Geometry check sheet. Reference: the model listing, model coordinates, mm. A direction names the side the tool comes from. Give positions to 0.01 mm unless a question says otherwise; leave off trailing zeros. Loops run counter-clockwise (first coordinate to the right, second up) from the corner with the lowest first, then second, coordinate; pieces in that order, holes last. Notation, with made-up numbers: (88, 0.5) -> (122, 0.5) arc R16 cw to (122, 4.5) -> close; hole circle Ø10 at (-26.5, 58.25). An arc over 180 degrees is marked (long way). Write item = value, one per line.
Autodesk Inventor part; units mm, degrees
ref_plane "YZ Plane" through (0, 0, 0) normal (1, 0, 0) x (0, 1, 0)
ref_plane "XZ Plane" through (0, 0, 0) normal (0, 1, 0) x (-1, 0, 0)
ref_plane "XY Plane" through (0, 0, 0) normal (0, 0, 1) x (1, 0, 0)
sketch "Skizze1" plane through (0, 0, 0) normal (0, 0, 1) x (1, 0, 0)
  circle A0 centre (0, 0) radius 4
  dimension "d0" = 8
extrude "Extrusion1" add sketch "Skizze1" along normal blind 40
sketch "Skizze2" plane through (0, 0, 0) normal (0, 0, -1) x (-1, 0, 0)
  circle A0 centre (0, 0) radius 3.5
  dimension "d3" = 7
extrude "Extrusion2" add sketch "Skizze2" along normal blind 5
thread "Gewinde1"
sketch "Skizze3" plane through (0, 0, 40) normal (0, 0, 1) x (1, 0, 0)
  circle A0 centre (0, 0) radius 3.5
  dimension "d8" = 7
extrude "Extrusion3" add sketch "Skizze3" along normal blind 7
properties part number "M8 inductive probe"
Item 1: Section check A-A, the plane y = 0. Record the cut outline in (x, z).
Answer:
outline = (-4, 0) -> (-3.5, 0) -> (-3.5, -5) -> (3.5, -5) -> (3.5, 0) -> (4, 0) -> (4, 40) -> (3.5, 40) -> (3.5, 47) -> (-3.5, 47) -> (-3.5, 40) -> (-4, 40) -> close
Item 2: Tool access check on faces 1 (the cylindrical face through (3.233, 1.341, 43.451)), 2 (the cylindrical face through (-3.233, 1.341, -2.465)), 3 (the cylindrical face through (-0.867, 3.905, 19.72)). Record the directions out of +Z, -Z, +X, -X, +Y, -Y that give a thin tool (end or side, any length) a straight path to the whole face; none if there is none.
Answer:
face_1 = +Z
face_2 = -Z
face_3 = +Z, -Z
Item 3: Section check C-C, the plane z = 29.5. Record the cut outline in (x, y), plus the area to 3 significant figures.
Answer:
outline = circle Ø8 at (0, 0)
area = 50.3 mm^2
Item 4: Section check D-D, the plane z = -1. Record the cut outline in (x, y), plus the area to 3 significant figures.
Answer:
outline = circle Ø7 at (0, 0)
area = 38.5 mm^2
Item 5: Gauge pin test, flat ends, axial feed: pin 1 (1.5 mm diameter, centred on x = 3, z = 26.5, fed in from +Y); pin 2 (1.5 mm diameter, centred on x = -3, y = 2.5, fed in from -Z); pin 3 (1.5 mm diameter, centred on y = -2.5, z = 2, fed in from -X); pin 4 (1.5 mm diameter, centred on y = -1.5, z = 8.5, fed in from -X). Record the tip position at first contact, or that the pin passes through.
Answer:
pin_1 = 3.31
pin_2 = -5
pin_3 = -3.6
pin_4 = -3.93
Item 6: Thickness scan on L1, parallel to Y at x = 0.25, z = 13; L2, parallel to Y at x = -2.25, z = 3; L3, parallel to X at y = 1.5, z = 30. Record the ranges inside material, lowest first. Write a range as [from, to].
Answer:
L1 = [-3.99, 3.99]
L2 = [-3.31, 3.31]
L3 = [-3.71, 3.71]
